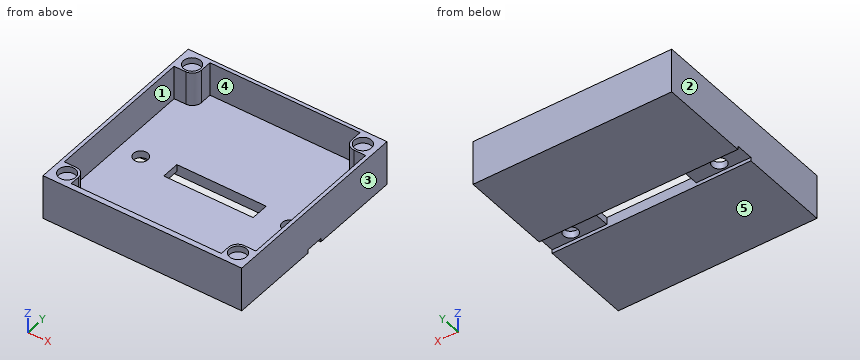
from build123d import *

# Parameters (mm, degrees)
SKICA1_W                 = 55.6
SKICA1_H                 = 55.6
P_IDAT_VYSUNUT_M2_DEPTH  = 3
SKICA4_W                 = 25
SKICA4_H                 = 5
ODEBRAT_VYSUNUT_M1_DEPTH = 2
SKICA5_W                 = 55.6
SKICA5_H                 = 5
ODEBRAT_VYSUNUT_M3_DEPTH = 1
SKICA14_W                = 53.6
SKICA14_H                = 1.5
P_IDAT_VYSUNUT_M9_DEPTH  = 9.5
SKICA17_R                = 2
ODEBRAT_VYSUNUT_M8_DEPTH = 4
SKICA19_W                = 6.8
SKICA19_H                = 6.8
P_IDAT_VYSUNUT_M10_DEPTH = 12.5
SKICA20_R                = 2.4
ODEBRAT_VYSUNUT_M9_DEPTH = 1.7
ZAOBLIT1_R               = 2.5


with BuildPart() as part:
    # Skica1 → Přidat vysunutím2 (new body)
    with BuildSketch(Plane.XY):
        Rectangle(SKICA1_W, SKICA1_H)
    extrude(amount=P_IDAT_VYSUNUT_M2_DEPTH)

    # Skica4 → Odebrat vysunutím1 (cut)
    with BuildSketch(Plane.XY.offset(3)):
        Rectangle(SKICA4_W, SKICA4_H)
    extrude(amount=-ODEBRAT_VYSUNUT_M1_DEPTH, mode=Mode.SUBTRACT)

    # Skica5 → Odebrat vysunutím3 (cut)
    with BuildSketch(Plane(origin=(0, 0, 0), x_dir=(-1, 0, 0), z_dir=(0, 0, -1))):
        Rectangle(SKICA5_W, SKICA5_H)
    extrude(amount=-ODEBRAT_VYSUNUT_M3_DEPTH, mode=Mode.SUBTRACT)

    # Skica14 → Přidat vysunutím9 (add)
    with BuildSketch(Plane.XY.offset(3)):
        Polygon((27.8, 27.8), (-27.8, 27.8), (-27.8, -27.8), (-26.8, -27.8), (-26.8, -26.8), (-26.8, -26.3), (-26.8, 26.8), (26.8, 26.8), (26.8, -26.3), (26.8, -27.8), (27.8, -27.8), align=None)
        with Locations((0, -27.05)):
            Rectangle(SKICA14_W, SKICA14_H)
    extrude(amount=P_IDAT_VYSUNUT_M9_DEPTH)

    # Skica17 → Odebrat vysunutím8 (cut)
    with BuildSketch(Plane(origin=(0, 0, 1), x_dir=(-1, 0, 0), z_dir=(0, 0, -1))):
        with Locations((-20.8, 0)):
            Circle(SKICA17_R)
        with Locations((20.8, 0)):
            Circle(SKICA17_R)
    extrude(amount=-ODEBRAT_VYSUNUT_M8_DEPTH, mode=Mode.SUBTRACT)

    # Skica19 → Přidat vysunutím10 (add)
    with BuildSketch(Plane(origin=(0, 0, 0), x_dir=(-1, 0, 0), z_dir=(0, 0, -1))):
        with Locations((-24.4, 24.4)):
            Rectangle(SKICA19_W, SKICA19_H)
        with Locations((24.4, 24.4)):
            Rectangle(SKICA19_W, SKICA19_H)
        with Locations((-24.4, -24.4)):
            Rectangle(SKICA19_W, SKICA19_H)
        with Locations((24.4, -24.4)):
            Rectangle(SKICA19_W, SKICA19_H)
    extrude(amount=-P_IDAT_VYSUNUT_M10_DEPTH)

    # Skica20 → Odebrat vysunutím9 (cut)
    with BuildSketch(Plane.XY.offset(12.5)):
        with Locations((-23.9, -23.9)):
            Circle(SKICA20_R)
        with Locations((-23.9, 23.9)):
            Circle(SKICA20_R)
        with Locations((23.900280565, 23.9)):
            Circle(SKICA20_R)
        with Locations((23.900280565, -23.9)):
            Circle(SKICA20_R)
    extrude(amount=-ODEBRAT_VYSUNUT_M9_DEPTH, mode=Mode.SUBTRACT)

    # Zaoblit1
    zaoblit1_edges = [part.edges().sort_by_distance(p)[0] for p in [
        (-21, 21, 7.75),
        (21, -21, 7.75),
        (-21, -21, 7.75),
        (21, 21, 7.75),
    ]]
    fillet(zaoblit1_edges, radius=ZAOBLIT1_R)


solid = part.part
Geometry check sheet. Reference: the model listing, model coordinates, mm. Face numbers are marked on the shaded views. A direction names the side the tool comes from. Give positions to 0.01 mm unless a question says otherwise; leave off trailing zeros. Write each loop counter-clockwise with the first axis right and the second up, starting at its lowest first coordinate (ties: lowest second). Pieces come first, ordered by that corner, then holes. Notation, with made-up numbers: M 23.25,54 L 54.25,54 A27 ccw 54.25,91 Z; hole C 9.5,89.5 d5. An arc over 180 degrees is marked long. Answer as CSV lines item,"result". Start each with the question number.
Q1. Release check for a two-part mould opening along X. For the marked faces 1, 2 and 3 record: pulls with the +X half, pulls with the -X half, needs draft (parallel to the pull), parting line crosses it, or undercut.
Q2. Tool access check on the marked faces 4 and 5. Record the directions out of +Z, -Z, +X, -X, +Y, -Y that give a thin tool (end or side, any length) a straight path to the whole face; none if there is none.
Q3. Go/stop test with flat-tipped pins: pin 1 (5 mm diameter, centred on x = 8, y = -9.5, fed in from -Z); pin 2 (2.5 mm diameter, centred on x = -24.5, y = 24, fed in from +Z); pin 3 (1 mm diameter, centred on x = -10, y = -16, fed in from +Z). Record where each tip stops, or that it passes through.
Q4. Material ranges on L1, parallel to Y at x = -24, z = 11.5; L2, parallel to Y at x = -12.5, z = 11.25; L3, parallel to X at y = 17.5, z = 3.75, recorded low to high.
Q5. Section check B-B, the plane z = 5. Record the cut outline in (x, y).
Q6. Section check C-C, the plane x = -15.5. Record the cut outline in (y, z).
Q7. Section check D-D, the plane z = 11.5. Record the cut outline in (x, y).
Q8. Section check A-A, the plane y = 0. Record the cut outline in (x, z).
Geometry says:
1,face 1,"undercut"
1,face 2,"pulls with the -X half"
1,face 3,"pulls with the +X half"
2,face 4,"+Z"
2,face 5,"-Z, +X, -X, +Y, -Y"
3,pin 1,"z = 0"
3,pin 2,"z = 10.8"
3,pin 3,"z = 3"
4,L1,"-27.8 to -26.3, -21.5 to -21, 21 to 21.5, 26.3 to 27.8"
4,L2,"-27.8 to -26.3, 26.8 to 27.8"
4,L3,"-27.8 to -26.8, 26.8 to 27.8"
5,outline,"M -27.8,-27.8 L 27.8,-27.8 L 27.8,27.8 L -27.8,27.8 Z; hole M -26.8,-21 L -23.5,-21 A2.5 cw -21,-23.5 L -21,-26.3 L 21,-26.3 L 21,-23.5 A2.5 cw 23.5,-21 L 26.8,-21 L 26.8,21 L 23.5,21 A2.5 cw 21,23.5 L 21,26.8 L -21,26.8 L -21,23.5 A2.5 cw -23.5,21 L -26.8,21 Z"
6,outline,"M -27.8,0 L -2.5,0 L -2.5,1 L 2.5,1 L 2.5,0 L 27.8,0 L 27.8,12.5 L 26.8,12.5 L 26.8,3 L -26.3,3 L -26.3,12.5 L -27.8,12.5 Z"
7,outline,"M -27.8,-27.8 L 27.8,-27.8 L 27.8,27.8 L -27.8,27.8 Z; hole M -26.8,-21 L -23.5,-21 A2.5 cw -21,-23.5 L -21,-26.3 L 21,-26.3 L 21,-23.5 A2.5 cw 23.5,-21 L 26.8,-21 L 26.8,21 L 23.5,21 A2.5 cw 21,23.5 L 21,26.8 L -21,26.8 L -21,23.5 A2.5 cw -23.5,21 L -26.8,21 Z; hole C -23.9,-23.9 d4.8; hole C -23.9,23.9 d4.8; hole C 23.9,-23.9 d4.8; hole C 23.9,23.9 d4.8"
8,outline,"M -27.8,1 L -22.8,1 L -22.8,3 L -26.8,3 L -26.8,12.5 L -27.8,12.5 Z; M -18.8,1 L -12.5,1 L -12.5,3 L -18.8,3 Z; M 12.5,1 L 18.8,1 L 18.8,3 L 12.5,3 Z; M 22.8,1 L 27.8,1 L 27.8,12.5 L 26.8,12.5 L 26.8,3 L 22.8,3 Z"
